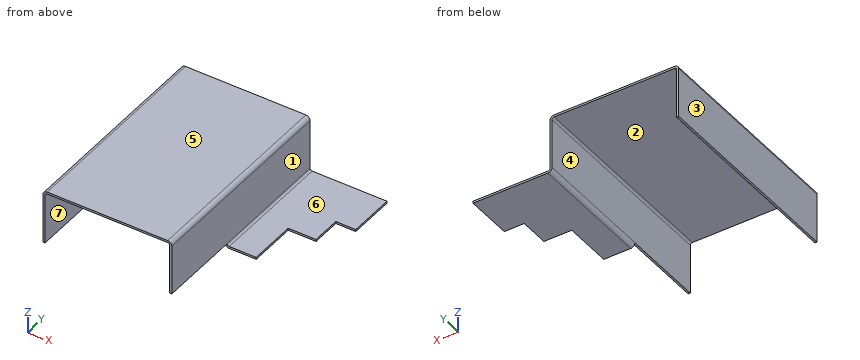
from build123d import *

# Parameters (mm, degrees)
Z_KLADN_PLECH1_DEPTH = 100
LEM_Z_HRANY1_DEPTH   = 60
OU_KO1_DEPTH         = 1


# Sheet-metal steps are written as plain solids
with BuildPart() as part:
    # Skica1 → Základní plech1 (new body)
    with BuildSketch(Plane(origin=(0, 0, 0), x_dir=(1, 0, 0), z_dir=(0, 1, 0))):
        with BuildLine():
            Line((0, 25), (0, 1))
            ThreePointArc((0, 1), (0.292893219, 0.292893219), (1, 0))
            Line((1, 0), (59, 0))
            ThreePointArc((59, 0), (59.707106781, 0.292893219), (60, 1))
            Line((60, 1), (60, 25))
            Line((60, 25), (61, 25))
            Line((61, 25), (61, 1))
            ThreePointArc((61, 1), (60.414213562, -0.414213562), (59, -1))
            Line((59, -1), (1, -1))
            ThreePointArc((1, -1), (-0.414213562, -0.414213562), (-1, 1))
            Line((-1, 1), (-1, 25))
            Line((-1, 25), (0, 25))
        make_face()
    extrude(amount=Z_KLADN_PLECH1_DEPTH)

    # Lem z hrany1 section (across the edge) → Lem z hrany1 (add)
    with BuildSketch(Plane(origin=(61, 40, -26), x_dir=(0, 0, 1), z_dir=(0, 1, 0))):
        with BuildLine():
            Line((-1, 1), (-1, 14))
            Line((-1, 14), (0, 14))
            Line((0, 14), (0, 1))
            ThreePointArc((0, 1), (0.292893219, 0.292893219), (1, 0))
            Line((1, 0), (1, -1))
            ThreePointArc((1, -1), (-0.414213562, -0.414213562), (-1, 1))
        make_face()
    extrude(amount=LEM_Z_HRANY1_DEPTH)

    # Skica9 → Ouško1 (add)
    with BuildSketch(Plane(origin=(0, 0, -27), x_dir=(-1, 0, 0), z_dir=(0, 0, -1))):
        Polygon((-98.025768087, 100), (-75, 100), (-75, 63.144926654), (-88.390120494, 63.144926654), (-88.390120494, 77.419960125), (-98.025768087, 77.419960125), align=None)
    extrude(amount=-OU_KO1_DEPTH)


solid = part.part
Model file for the job. Use its own axes, mm. Face numbers are marked on the shaded views. A direction names the side the tool comes from. Give positions to 0.01 mm unless a question says otherwise; leave off trailing zeros. Loops run counter-clockwise (first coordinate to the right, second up) from the corner with the lowest first, then second, coordinate; pieces in that order, holes last.
Item 1: Mould opens along X. For the marked faces 1, 2, 3 and 4 say: +X half, -X half, draft (parallel to the pull), parting line (faces both ways), or undercut.
Check values:
face 1: +X half
face 2: undercut
face 3: -X half
face 4: undercut
Item 2: Slice it at B-B (y = 49.5). Write the cut outline in (x, z).
Check values:
outline: (-1, -25) - (0, -25) - (0, -1) arc R1 cw to (1, 0) - (59, 0) arc R1 cw to (60, -1) - (60, -25) arc R2 ccw to (62, -27) - (75, -27) - (75, -26) - (62, -26) arc R1 cw to (61, -25) - (61, -1) arc R2 ccw to (59, 1) - (1, 1) arc R2 ccw to (-1, -1) - close
Item 3: Which spindle directions (+Z, -Z, +X, -X, +Y, -Y) get a long thin tool onto all of the face, cutting with end or side? Do the marked faces 5, 6 and 7. Say none if no direction does.
Check values:
face 5: +Z, +X, -X, +Y, -Y
face 6: +Z, +X, +Y, -Y
face 7: -Z, +Y, -Y
Item 4: Slice it at D-D (x = 77.5). Write the cut outline in (y, z).
Check values:
outline: (63.14, -27) - (100, -27) - (100, -26) - (63.14, -26) - close
Item 5: Drill centre lines: line 1 along X through (y, z) = (51.5, -2.5); line 2 along Z through (x, y) = (23, 44.5); line 3 along Z through (x, y) = (75.5, 88). Where is each one in solid material? Low to high.
Check values:
line 1: x = -1 to 0, 60 to 61
line 2: z = 0 to 1
line 3: z = -27 to -26
Item 6: Slice it at A-A (z = -18.5). Write the cut outline in (x, y).
Check values:
outline: (-1, 0) - (0, 0) - (0, 100) - (-1, 100) - close; (60, 0) - (61, 0) - (61, 100) - (60, 100) - close
Item 7: Slice it at C-C (y = 69). Write the cut outline in (x, z), plus the area to 3 significant figures.
Check values:
outline: (-1, -25) - (0, -25) - (0, -1) arc R1 cw to (1, 0) - (59, 0) arc R1 cw to (60, -1) - (60, -25) arc R2 ccw to (62, -27) - (88.39, -27) - (88.39, -26) - (62, -26) arc R1 cw to (61, -25) - (61, -1) arc R2 ccw to (59, 1) - (1, 1) arc R2 ccw to (-1, -1) - close
area: 139 mm2
Item 8: Drop flat-ended pins along their axis: P1, Ø2, axis at x = 71, z = -26, coming from the -Y side; P2, Ø0.8, axis at x = -0.5, y = 41, coming from the -Z side; P3, Ø3, axis at y = 12, z = -13, coming from the +X side. Give the stop position or say it passes through.
Check values:
P1: stops at y = 40
P2: stops at z = -25
P3: stops at x = 61
